from build123d import *

# Parameters (mm, degrees)
BOSS_EXTRUDE1_DEPTH       = 1
BOSS_EXTRUDE2_DEPTH       = 5
BOSS_EXTRUDE3_DEPTH       = 5
CUT_EXTRUDE3_DEPTH        = 10
CUT_EXTRUDE2_DEPTH        = 10
TAP_DRILL_FOR_3_56_TAP1_D = 2.0828
SKETCH29_W                = 25
SKETCH29_H                = 1.864988104
CUT_EXTRUDE4_DEPTH        = 10


with BuildPart() as part:
    # Sketch2 → Boss-Extrude1 (new body)
    with BuildSketch(Plane.XY):
        with BuildLine():
            Line((-33.5, 46), (33.5, 46))
            ThreePointArc((33.5, 46), (34.560660172, 45.560660172), (35, 44.5))
            Line((35, 44.5), (35, -44.5))
            ThreePointArc((35, -44.5), (34.560660172, -45.560660172), (33.5, -46))
            Line((33.5, -46), (-33.5, -46))
            ThreePointArc((-33.5, -46), (-34.560660172, -45.560660172), (-35, -44.5))
            Line((-35, -44.5), (-35, 44.5))
            ThreePointArc((-35, 44.5), (-34.560660172, 45.560660172), (-33.5, 46))
        make_face()
    extrude(amount=BOSS_EXTRUDE1_DEPTH)

    # Sketch3 → Boss-Extrude2 (add)
    with BuildSketch(Plane.XY.offset(1)):
        with BuildLine():
            Line((-32, 44.5), (-32, -44.5))
            ThreePointArc((-32, -44.5), (-33.5, -46), (-35, -44.5))
            Line((-35, -44.5), (-35, 44.5))
            ThreePointArc((-35, 44.5), (-33.5, 46), (-32, 44.5))
        make_face()
        with BuildLine():
            Line((32, 44.5), (32, -44.5))
            ThreePointArc((32, -44.5), (33.5, -46), (35, -44.5))
            Line((35, -44.5), (35, 44.5))
            ThreePointArc((35, 44.5), (33.5, 46), (32, 44.5))
        make_face()
    extrude(amount=BOSS_EXTRUDE2_DEPTH)

    # Sketch4 → Boss-Extrude3 (add)
    with BuildSketch(Plane.XY.offset(1)):
        with BuildLine():
            Line((-33.5, 46), (33.5, 46))
            ThreePointArc((33.5, 46), (35, 44.5), (33.5, 43))
            Line((33.5, 43), (-33.5, 43))
            ThreePointArc((-33.5, 43), (-35, 44.5), (-33.5, 46))
        make_face()
        with BuildLine():
            Line((-33.5, -46), (33.5, -46))
            ThreePointArc((33.5, -46), (35, -44.5), (33.5, -43))
            Line((33.5, -43), (-33.5, -43))
            ThreePointArc((-33.5, -43), (-35, -44.5), (-33.5, -46))
        make_face()
    extrude(amount=BOSS_EXTRUDE3_DEPTH)

    # Sketch5 → Cut-Extrude3 (cut)
    with BuildSketch(Plane(origin=(0, 46, 0), x_dir=(1, 0, 0), z_dir=(0, 1, 0))):
        with BuildLine():
            ThreePointArc((-14.89567412, -5.42869642), (-15.182613275, -5.338166714), (-15.36564636, -5.099360107))
            Line((-15.36564636, -5.099360107), (-16.066024836, -3.170663686))
            ThreePointArc((-16.066024836, -3.170663686), (-16.088488439, -3.0866426), (-16.096052596, -3))
            Line((-16.096052596, -3), (-16.096052596, -1.612708973))
            ThreePointArc((-16.096052596, -1.612708973), (-15.949605986, -1.259155582), (-15.596052596, -1.112708973))
            Line((-15.596052596, -1.112708973), (-8.896052596, -1.112708973))
            ThreePointArc((-8.896052596, -1.112708973), (-8.542499205, -1.259155582), (-8.396052596, -1.612708973))
            Line((-8.396052596, -1.612708973), (-8.396052596, -3))
            ThreePointArc((-8.396052596, -3), (-8.403616752, -3.0866426), (-8.426080356, -3.170663686))
            Line((-8.426080356, -3.170663686), (-9.126458831, -5.099360107))
            ThreePointArc((-9.126458831, -5.099360107), (-9.309491917, -5.338166714), (-9.596431071, -5.42869642))
            Line((-9.596431071, -5.42869642), (-14.89567412, -5.42869642))
        make_face()
    extrude(amount=-CUT_EXTRUDE3_DEPTH, mode=Mode.SUBTRACT)

    # Sketch7 → Cut-Extrude2 (cut)
    with BuildSketch(Plane(origin=(0, 0, 0), x_dir=(-1, 0, 0), z_dir=(0, 0, -1))):
        with BuildLine():
            Line((-19.322853535, -9.222931336), (-9.322853535, -9.222931336))
            ThreePointArc((-9.322853535, -9.222931336), (-8.615746754, -9.515824554), (-8.322853535, -10.222931336))
            Line((-8.322853535, -10.222931336), (-8.322853535, -33.222931336))
            ThreePointArc((-8.322853535, -33.222931336), (-8.615746754, -33.930038117), (-9.322853535, -34.222931336))
            Line((-9.322853535, -34.222931336), (-19.322853535, -34.222931336))
            ThreePointArc((-19.322853535, -34.222931336), (-20.029960316, -33.930038117), (-20.322853535, -33.222931336))
            Line((-20.322853535, -33.222931336), (-20.322853535, -10.222931336))
            ThreePointArc((-20.322853535, -10.222931336), (-20.029960316, -9.515824554), (-19.322853535, -9.222931336))
        make_face()
    extrude(amount=-CUT_EXTRUDE2_DEPTH, mode=Mode.SUBTRACT)

    # Tap Drill for #3-56 Tap1 (through all)
    with Locations(Plane.XY.offset(6)):
        with Locations((-33.5, 44.5), (-33.5, 0), (-33.5, -44.5), (33.5, -44.5), (33.499705774, 0), (33.5, 44.5)):
            Hole(TAP_DRILL_FOR_3_56_TAP1_D / 2)

    # Sketch29 → Cut-Extrude4 (cut)
    with BuildSketch(Plane(origin=(0, 46, 0), x_dir=(1, 0, 0), z_dir=(0, 1, 0))):
        with Locations((10.342588325, -5.067505948)):
            Rectangle(SKETCH29_W, SKETCH29_H)
    extrude(amount=-CUT_EXTRUDE4_DEPTH, mode=Mode.SUBTRACT)


solid = part.part
Geometry: final body of the model. Coordinates: model frame, mm. A direction names the side the tool comes from. Round coordinates to 2 decimals unless told otherwise and drop trailing zeros. Order: outer loops, then holes, each group sorted by start corner. A loop starts at its lowest first (then second) coordinate and runs counter-clockwise, first axis right, second up. Notation, with made-up numbers: (24.25, 26) -> (35.25, 26) arc R23 ccw to (35.25, 56) -> close; hole circle Ø2 at (32, -17.5). An arc over 180 degrees is marked (long way). Put each result on its own line as item: value. Start each with the question number.
Q1. Section C-C on x = -28.5. Return the cut outline in (y, z).
Q2. Line query: probe 1 along Y at (x, z) = (33.5, 3.75); probe 2 along X at (y, z) = (-19.5, 5.2); probe 3 along Y at (x, z) = (-23, 3.45). Output: solid intervals per line, ascending.
Q3. Section B-B on x = 13. Return the cut outline in (y, z).
Q4. First-contact query: pin 1 (0.7 mm diameter, centred on y = 45, z = 2, fed in from -X); pin 2 (2 mm diameter, centred on x = 2, y = 24, fed in from +Z); pin 3 (1.9 mm diameter, centred on x = 33.5, y = 0, fed in from -Z). Flat tips, straight axial feed; report the tip coordinate or a pass-through.
Q5. Section A-A on y = -20.5. Return the cut outline in (x, z), and give its area (3 significant figures).
Q6. Reachability of faces 1 (the flat face through (22.843, 45, 5)), 2 (the flat face through (0, -43, 3)), 3 (the flat face through (-12, 45, 5.429)), 4 (the flat face through (-35, -1, 3)), 5 (the cylindrical face through (-33.981, -45.424, 2.958)) from +Z, -Z, +X, -X, +Y, -Y: full face, straight path, thin tool, end or side. Return the list, or none.
Q7. Pull-direction query (Z, two-part tool) for faces 6 (the flat face through (10, 45, 4.135)), 7 (the flat face through (32, 1, 3)), 8 (the flat face through (-15.71, 44.52, 4.15)); classes: +Z half, -Z half, draft (parallel to the pull), parting line (faces both ways), or undercut.
Q8. Section D-D on y = 13. Return the cut outline in (x, z), and give its area (3 significant figures).
Ans:
1. outline: (-46, 0) -> (46, 0) -> (46, 6) -> (43, 6) -> (43, 1) -> (-43, 1) -> (-43, 6) -> (-46, 6) -> close
2. probe 1: y = -46 to -45.54, -43.46 to -1.04, 1.04 to 43.46, 45.54 to 46
2. probe 2: x = -35 to -32, 32 to 35
2. probe 3: y = -46 to -43, 43 to 46
3. outline: (-46, 0) -> (-34.22, 0) -> (-34.22, 1) -> (-43, 1) -> (-43, 6) -> (-46, 6) -> close; (-9.22, 0) -> (46, 0) -> (46, 4.14) -> (43, 4.14) -> (43, 1) -> (-9.22, 1) -> close
4. pin 1: stops at x = -34.99
4. pin 2: stops at z = 1
4. pin 3: passes through
5. outline: (-35, 0) -> (8.32, 0) -> (8.32, 1) -> (-32, 1) -> (-32, 6) -> (-35, 6) -> close; (20.32, 0) -> (35, 0) -> (35, 6) -> (32, 6) -> (32, 1) -> (20.32, 1) -> close
5. area: 88.0 mm2
6. face 1: +Z, +Y
6. face 2: +Z
6. face 3: +Y
6. face 4: +Z, -Z, -X, +Y, -Y
6. face 5: +Z, -Z
7. face 6: +Z half
7. face 7: draft
7. face 8: undercut
8. outline: (-35, 0) -> (35, 0) -> (35, 6) -> (32, 6) -> (32, 1) -> (-32, 1) -> (-32, 6) -> (-35, 6) -> close
8. area: 100 mm2
